Check sheet for the drawn part. Datum: minimum x, y, z corner. Units: mm. A direction names the side the tool comes from. Round coordinates to 2 decimals unless told otherwise and drop trailing zeros. Write each loop counter-clockwise with the first axis right and the second up, starting at its lowest first coordinate (ties: lowest second). Pieces come first, ordered by that corner, then holes. Notation, with made-up numbers: M 16.5,-38.75 L 20.5,-38.75 A21 ccw 20.5,-20.75 Z; hole C 63.25,-8 d11. An arc over 180 degrees is marked long. One line per item, written item: value. Start each with the question number.
1. Access from +Z, -Z, +X, -X, +Y, -Y to the whole of each face (thin tool, end or side, straight path). Record for the marked faces 1, 2 and 3.
2. Release check for a two-part mould opening along Z. For the marked faces 4, 5 and 6 record: pulls with the +Z half, pulls with the -Z half, needs draft (parallel to the pull), parting line crosses it, or undercut.
3. Section check A-A (x = 304.5). Record the boundary of the cut face in (y, z).
4. Section check D-D (y = 853). Record the boundary of the cut face in (x, z).
5. Depth check by flat-ended pin: P1, Ø1, axis at x = 717.5, y = 732, coming from the +Z side. Enter the tip coordinate at first touch or a pass-through.
6. Section check C-C (y = 167.5). Record the boundary of the cut face in (x, z).
7. Scan lines: probe 1 along X at (y, z) = (319, 291); probe 2 along Z at (x, y) = (937.5, 736); probe 3 along Z at (x, y) = (1194.5, 421.5). Record each from-to range of solid material in increasing order. Write a range as [from, to].
8. Section check B-B (z = 908). Record the boundary of the cut face in (x, y).
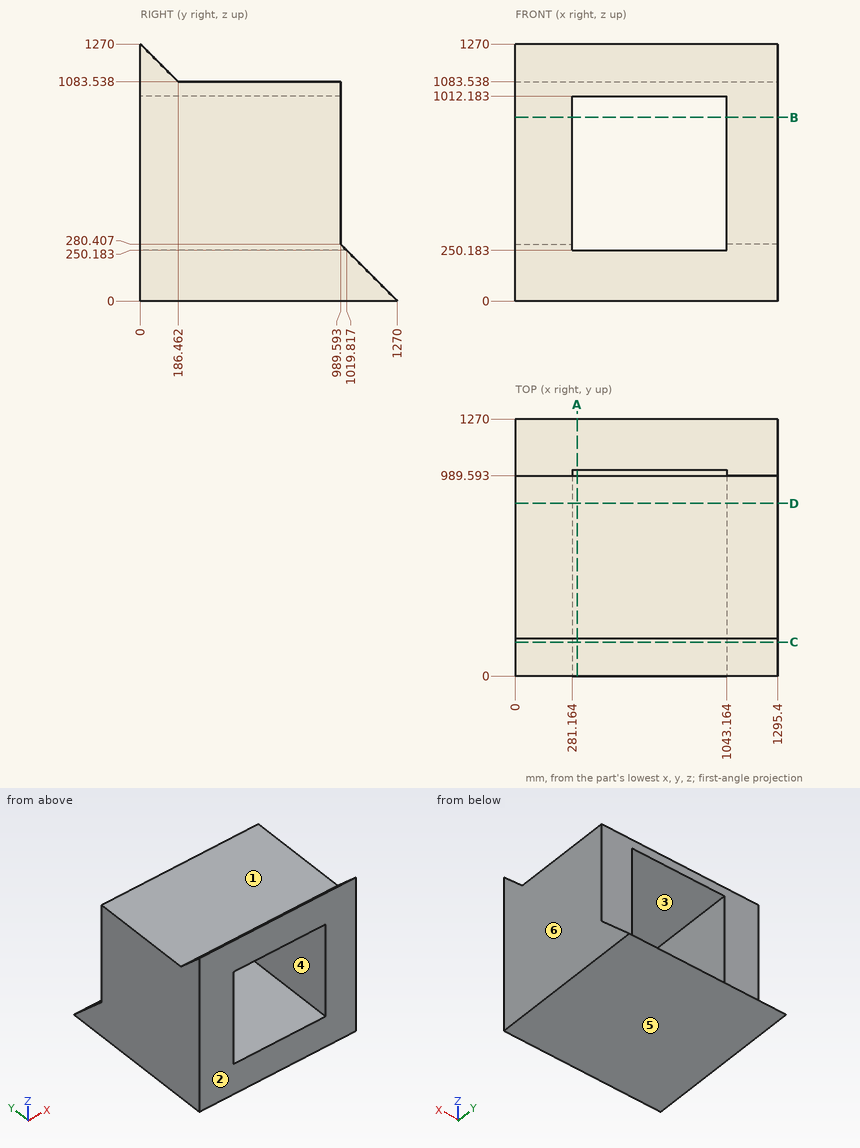
Result sheet:
1. face 1: +Z, +X, -X, +Y
1. face 2: +Z, -Z, +X, -X, -Y
1. face 3: +Y, -Y
2. face 4: undercut
2. face 5: pulls with the -Z half
2. face 6: needs draft
3. outline: M 0,0 L 1270,0 L 1019.82,250.18 L 0,250.18 Z; M 0,1012.18 L 989.59,1012.18 L 989.59,1083.54 L 186.46,1083.54 L 0,1270 Z
4. outline: M 0,0 L 1295.4,0 L 1295.4,1083.54 L 0,1083.54 Z; hole M 281.16,250.18 L 1043.16,250.18 L 1043.16,1012.18 L 281.16,1012.18 Z
5. P1: stops at z = 1083.54
6. outline: M 0,0 L 1295.4,0 L 1295.4,1102.5 L 0,1102.5 Z; hole M 281.16,250.18 L 1043.16,250.18 L 1043.16,1012.18 L 281.16,1012.18 Z
7. probe 1: x = [0, 281.16], [1043.16, 1295.4]
7. probe 2: z = [0, 250.18], [1012.18, 1083.54]
7. probe 3: z = [0, 1083.54]
8. outline: M 0,0 L 281.16,0 L 281.16,989.59 L 0,989.59 Z; M 1043.16,0 L 1295.4,0 L 1295.4,989.59 L 1043.16,989.59 Z
